from build123d import *

# Parameters (mm, degrees)
SKETCH1_W           = 496
SKETCH1_H           = 40
SKETCH1_R           = 5.5
SKETCH1_R_2         = 3.6
BOSS_EXTRUDE1_DEPTH = 5
SKETCH2_R           = 6.5
CUT_EXTRUDE1_DEPTH  = 3
FILLET1_R           = 10


with BuildPart() as part:
    # Sketch1 → Boss-Extrude1 (new body)
    with BuildSketch(Plane(origin=(0, 0, 0), x_dir=(1, 0, 0), z_dir=(0, 1, 0))):
        with Locations((-144.299026304, 43.778006447)):
            Rectangle(SKETCH1_W, SKETCH1_H)
        with Locations(Location((-379.799026304, 53.278006447, 0), (0, 0, 270))):
            Circle(SKETCH1_R, mode=Mode.SUBTRACT)
        with Locations(Location((91.200973696, 52.778006447, 0), (0, 0, 270))):
            Circle(SKETCH1_R, mode=Mode.SUBTRACT)
        with Locations(Location((-293.099026304, 56.844673113, 0), (0, 0, 270))):
            Circle(SKETCH1_R_2, mode=Mode.SUBTRACT)
        with Locations(Location((-193.899026304, 56.844673113, 0), (0, 0, 270))):
            Circle(SKETCH1_R_2, mode=Mode.SUBTRACT)
        with Locations(Location((-94.699026304, 56.844673113, 0), (0, 0, 270))):
            Circle(SKETCH1_R_2, mode=Mode.SUBTRACT)
        with Locations(Location((4.500973696, 56.844673113, 0), (0, 0, 270))):
            Circle(SKETCH1_R_2, mode=Mode.SUBTRACT)
        with Locations(Location((-144.299026304, 56.844673113, 0), (0, 0, 270))):
            Circle(SKETCH1_R_2, mode=Mode.SUBTRACT)
    extrude(amount=BOSS_EXTRUDE1_DEPTH)

    # Sketch2 → Cut-Extrude1 (cut)
    with BuildSketch(Plane.XZ):
        with Locations(Location((-379.799026304, -53.278006447, 0), (0, 0, 270))):
            Circle(SKETCH2_R)
        with Locations(Location((91.200973696, -52.778006447, 0), (0, 0, 270))):
            Circle(SKETCH2_R)
    extrude(amount=-CUT_EXTRUDE1_DEPTH, mode=Mode.SUBTRACT)

    # Fillet1
    fillet1_edges = [part.edges().sort_by_distance(p)[0] for p in [
        (-392.299026304, 2.5, -63.778006447),
        (103.700973696, 2.5, -63.778006447),
    ]]
    fillet(fillet1_edges, radius=FILLET1_R)


solid = part.part
Here's how the part is built. I have some questions about the finished solid (model axes, mm). A direction names the side the tool comes from. Round coordinates to 2 decimals unless told otherwise and drop trailing zeros. Order: outer loops, then holes, each group sorted by start corner. A loop starts at its lowest first (then second) coordinate and runs counter-clockwise, first axis right, second up. Notation, with made-up numbers: M 43,17 L 84,17 A8 cw 84,29 Z; hole C -30,-9.75 d1. An arc over 180 degrees is marked long. One line per question, with ' | ' between items.
1) I need wall thicknesses on line 1 (X direction, y = 2.6, z = -51.5); line 2 (X direction, y = 3.6, z = -50); line 3 (Z direction, x = -293, y = 1.7). Which ranges of each line are inside material? Lowest first, please.
Checked values:
line 1: x = -392.3 to -386.05, -373.55 to 84.83, 97.57 to 103.7 | line 2: x = -392.3 to -384.22, -375.38 to 86.45, 95.95 to 103.7 | line 3: z = -63.78 to -60.44, -53.25 to -23.78
2) Imagine slicing it at A-A, the plane y = 3.8. Write out the boundary of the cut face in (x, z), plus the area to 3 significant figures.
Checked values:
outline: M -392.3,-53.78 A10 ccw -382.3,-63.78 L 93.7,-63.78 A10 ccw 103.7,-53.78 L 103.7,-23.78 L -392.3,-23.78 Z; hole C -379.8,-53.28 d11; hole C -293.1,-56.84 d7.2; hole C -193.9,-56.84 d7.2; hole C -144.3,-56.84 d7.2; hole C -94.7,-56.84 d7.2; hole C 4.5,-56.84 d7.2; hole C 91.2,-52.78 d11 | area: 19,400 mm²
3) I'm going to push flat-ended pins straight in: pin 1 Ø6.5 at (x, z) = (4.5, -56.84) entering from -Y; pin 2 Ø10.5 at (x, z) = (-380.5, -53.5) entering from -Y. Where does each tip first touch, or does it pass through?
Checked values:
pin 1: passes through | pin 2: stops at y = 3
4) We'd pull the mould along Z, two halves only. Please class faces 3 (the flat face through (-148, 0, -44)), 4 (the flat face through (-374, 3, -55)), 5 (the cylindrical face through (100.69, 2.54, -60.93)): released by +Z, released by -Z, zero draft, split by the parting line, or undercut.
Checked values:
face 3: zero draft | face 4: undercut | face 5: released by -Z
5) On a 3-axis mill with a long thin cutter (end or side, diameter ignored), from which of +Z, -Z, +X, -X, +Y, -Y can I reach the whole of each face in a straight line? I mean faces 1 (the cylindrical face through (87.85, 3.99, -57.14)), 2 (the flat face through (93, 3, -47)). Say none if no direction works.
Checked values:
face 1: +Y, -Y | face 2: -Y
